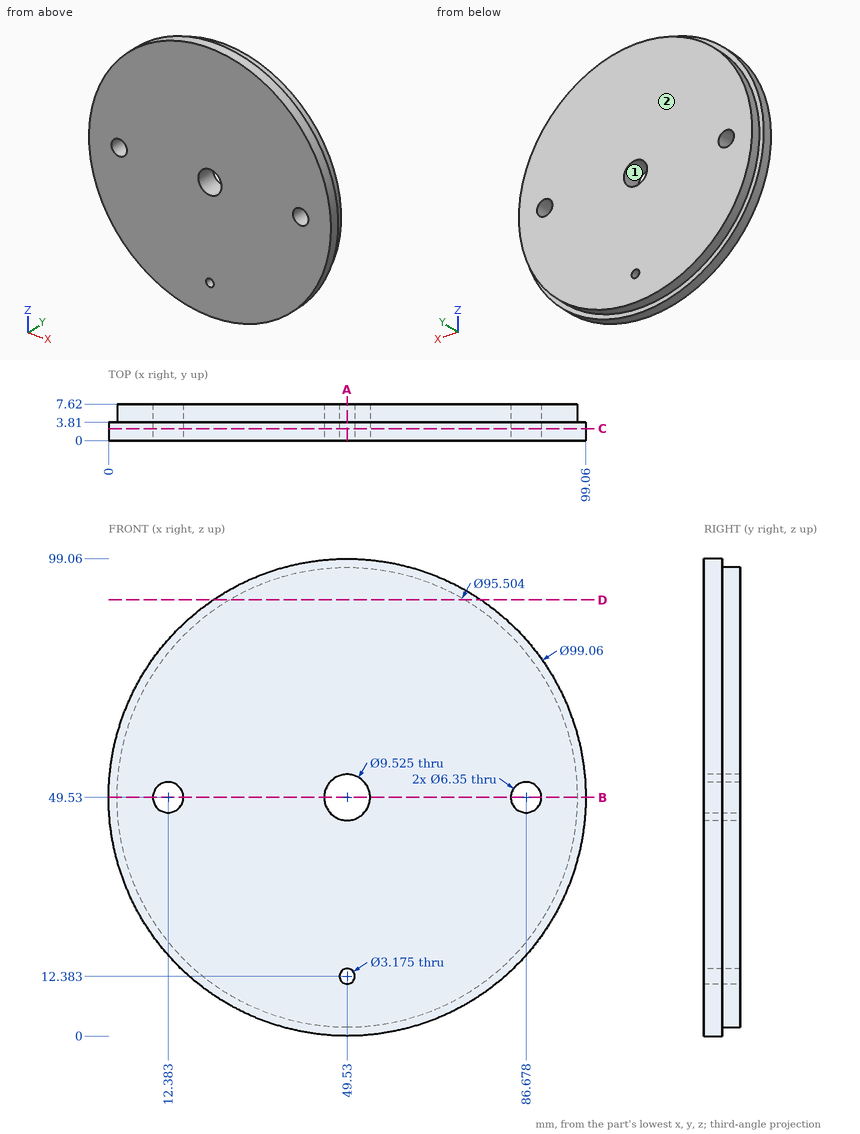
Verification items for this drawing (mm, ordinates from the low corner). Give positions to 0.01 mm unless a question says otherwise; leave off trailing zeros. Write each loop counter-clockwise with the first axis right and the second up, starting at its lowest first coordinate (ties: lowest second). Pieces come first, ordered by that corner, then holes. Notation, with made-up numbers: (73, 31) -> (83, 31) arc R35 cw to (83, 64) -> close; hole circle Ø10 at (17, 70.5). An arc over 180 degrees is marked (long way). Use CSV: the item, a comma, the result in double quotes. Start each with the question number.
Q1. Scan lines: line 1 along X through (y, z) = (3.5, 49.53); line 2 along X through (y, z) = (0.5, 51.5) (1 decimal); line 3 along Z through (x, y) = (84, 1) (1 decimal). Record each from-to range of solid material in increasing order.
Q2. Cross-section at C-C on y = 2.5. Count the separate pieces of the cut face and the enclosed holes in it, and give its area (3 significant figures).
Q3. Cross-section at B-B on z = 49.53. Enter the section's corners in (x, y).
Q4. Cross-section at D-D on z = 90.5. Enter the section's corners in (x, y).
Q5. Cross-section at A-A on x = 49.53. Enter the section's corners in (y, z) (1 decimal).
Q6. Release check for a two-part mould opening along X. For the marked faces 1 and 2 record: +X half, -X half, draft (parallel to the pull), parting line (faces both ways), or undercut.
Q7. Depth check by flat-ended pin: P1, Ø1.5, axis at y = 3, z = 15, coming from the -X side (1 decimal); P2, Ø2, axis at y = 6, z = 66, coming from the -X side; P3, Ø1.5, axis at y = 6.5, z = 45, coming from the +X side. Enter the tip coordinate at first touch or a pass-through.
Working result:
1,line 1,"x = 0 to 9.21, 15.56 to 44.77, 54.29 to 83.5, 89.85 to 99.06"
1,line 2,"x = 0 to 9.9, 14.9 to 45.2, 53.9 to 84.2, 89.2 to 99"
1,line 3,"z = 14 to 47.8, 51.2 to 85.1"
2,separate pieces,"1"
2,enclosed holes,"4"
2,area,"7,560 mm^2"
3,outline,"(0, 0) -> (9.21, 0) -> (9.21, 7.62) -> (1.78, 7.62) -> (1.78, 3.81) -> (0, 3.81) -> close; (15.56, 0) -> (44.77, 0) -> (44.77, 7.62) -> (15.56, 7.62) -> close; (54.29, 0) -> (83.5, 0) -> (83.5, 7.62) -> (54.29, 7.62) -> close; (89.85, 0) -> (99.06, 0) -> (99.06, 3.81) -> (97.28, 3.81) -> (97.28, 7.62) -> (89.85, 7.62) -> close"
4,outline,"(21.7, 0) -> (77.36, 0) -> (77.36, 3.81) -> (74.06, 3.81) -> (74.06, 7.62) -> (25, 7.62) -> (25, 3.81) -> (21.7, 3.81) -> close"
5,outline,"(0, 0) -> (3.8, 0) -> (3.8, 1.8) -> (7.6, 1.8) -> (7.6, 10.8) -> (0, 10.8) -> close; (0, 14) -> (7.6, 14) -> (7.6, 44.8) -> (0, 44.8) -> close; (0, 54.3) -> (7.6, 54.3) -> (7.6, 97.3) -> (3.8, 97.3) -> (3.8, 99.1) -> (0, 99.1) -> close"
6,face 1,"undercut"
6,face 2,"draft"
7,P1,"stops at x = 13.3"
7,P2,"stops at x = 4.35"
7,P3,"stops at x = 97.13"
